from build123d import *

# Parameters (mm, degrees)
F1_DEPTH     = 6
F2_R         = 0.975
F3_DEPTH     = 6.001
F4_T1_DEPTH  = 6
F4_T3_DEPTH  = 6
F4_T5_DEPTH  = 13.5
F4_T7_DEPTH  = 13.5
F4_T9_DEPTH  = 13.5
F4_T11_DEPTH = 13.5
F4_T13_DEPTH = 13.4624057783
F5_SIZE      = 0.5


# Not quite as in the source:
# - a fillet or chamfer that OpenCascade refuses, or shapes differently, is made with other operations: its cross-section is extruded or revolved along the edge and cut away or added


with BuildPart() as f1:
    # F0 (on Top) → F1 (new body)
    with BuildSketch(Plane.XY):
        Polygon((0, 1.9), (0, 0), (1.35, 0), (1.35, 11.3), (-7.85, 11.3), (-7.85, 7.55), (-4.85, 7.55), (-4.85, 0), (-3.5, 0), (-3.5, 8.5), (0, 8.5), align=None)
        Polygon((-0.9, 0), (0, 0), (0, 1.9), (-0.9, 1), align=None)
    extrude(amount=F1_DEPTH)

    # F2 (on face) → F3 (cut, through all)
    with BuildSketch(Plane.XY.offset(6)):
        with Locations((-5.8098790534, 9.425)):
            Circle(F2_R)
    extrude(amount=-F3_DEPTH, mode=Mode.SUBTRACT)

    # F4: fillet of radius 1.5 on 7 edges, made by hand

    # F4_s2 → F4_t1 (join)
    with BuildSketch(Plane.XY):
        with BuildLine():
            ThreePointArc((0, 7), (-0.4393398282, 8.0606601718), (-1.5, 8.5))
            Line((-1.5, 8.5), (0, 8.5))
            Line((0, 8.5), (0, 7))
        make_face()
    extrude(amount=F4_T1_DEPTH)

    # F4_s4 → F4_t3 (join)
    with BuildSketch(Plane.XY):
        with BuildLine():
            ThreePointArc((-2, 8.5), (-3.0606601718, 8.0606601718), (-3.5, 7))
            Line((-3.5, 7), (-3.5, 8.5))
            Line((-3.5, 8.5), (-2, 8.5))
        make_face()
    extrude(amount=F4_T3_DEPTH)

    # F4_s6 → F4_t5 (cut)
    with BuildSketch(Plane.XY.offset(-3.75)):
        with BuildLine():
            ThreePointArc((1.35, 1.5), (0.9106601718, 0.4393398282), (-0.15, 0))
            Line((-0.15, 0), (1.35, 0))
            Line((1.35, 0), (1.35, 1.5))
        make_face()
    extrude(amount=F4_T5_DEPTH, mode=Mode.SUBTRACT)

    # F4_s8 → F4_t7 (cut)
    with BuildSketch(Plane.XY.offset(-3.75)):
        with BuildLine():
            ThreePointArc((1.35, 9.8), (0.9106601718, 10.8606601718), (-0.15, 11.3))
            Line((-0.15, 11.3), (1.35, 11.3))
            Line((1.35, 11.3), (1.35, 9.8))
        make_face()
    extrude(amount=F4_T7_DEPTH, mode=Mode.SUBTRACT)

    # F4_s10 → F4_t9 (cut)
    with BuildSketch(Plane.XY.offset(-3.75)):
        with BuildLine():
            ThreePointArc((-7.85, 9.8), (-7.4106601718, 10.8606601718), (-6.35, 11.3))
            Line((-6.35, 11.3), (-7.85, 11.3))
            Line((-7.85, 11.3), (-7.85, 9.8))
        make_face()
    extrude(amount=F4_T9_DEPTH, mode=Mode.SUBTRACT)

    # F4_s12 → F4_t11 (cut)
    with BuildSketch(Plane.XY.offset(-3.75)):
        with BuildLine():
            ThreePointArc((-6.35, 7.55), (-7.4106601718, 7.9893398282), (-7.85, 9.05))
            Line((-7.85, 9.05), (-7.85, 7.55))
            Line((-7.85, 7.55), (-6.35, 7.55))
        make_face()
    extrude(amount=F4_T11_DEPTH, mode=Mode.SUBTRACT)

    # F4_s14 → F4_t13 (cut)
    with BuildSketch(Plane.XY.offset(-3.7312028891)):
        with BuildLine():
            ThreePointArc((-3.5, 0), (-4.4624297731, 0.4862505658), (-4.85, 1.4924811557))
            Line((-4.85, 1.4924811557), (-4.85, 0))
            Line((-4.85, 0), (-3.5, 0))
        make_face()
    extrude(amount=F4_T13_DEPTH, mode=Mode.SUBTRACT)

    # F5
    f5_edges = [f1.edges().sort_by_distance(p)[0] for p in [
        (-6.784879, 9.425, 6),
        (-6.784879, 9.425, 0),
    ]]
    chamfer(f5_edges, length=F5_SIZE)


solid = f1.part
Can you work these out from the model? Positions are in its coordinate system, mm. A direction names the side the tool comes from. Round coordinates to 2 decimals unless told otherwise and drop trailing zeros. Loops run counter-clockwise (first coordinate to the right, second up) from the corner with the lowest first, then second, coordinate; pieces in that order, holes last. Notation, with made-up numbers: (2.25, 11) - (41.25, 11) arc R19 cw to (41.25, 35) - close; hole circle Ø10 at (47.5, 22). An arc over 180 degrees is marked (long way). Answer in a Markdown table with one row per item. Add a question column.
Q1. For pin 1 Ø1.2 at (x, z) = (-6, 2) entering from -Y; pin 2 Ø1.2 at (x, y) = (-5.81, 9.43) entering from -Z; pin 3 Ø1 at (x, z) = (-2.5, 3.5) entering from -Y; pin 4 Ø3 at (y, z) = (3.5, 2.5) entering from -X, each with a flat end and sliding along its axis, tell me the tip position at first contact or that it passes through.
Q2. We'd pull the mould along X, two halves only. Please class faces 1 (the cylindrical face through (-3.05, 8.07, 2.96)), 2 (the flat face through (-3.5, 3, 3)), 3 (the flat face through (-4.85, 5, 3)), 4 (the flat face through (-3.2, 8.2, 6)): pulls with the +X half, pulls with the -X half, needs draft (parallel to the pull), parting line crosses it, or undercut.
Q3. I want a section at B-B on z = 3.45. List the corners of the cut face in (x, y) for me (3 decimals).
Q4. I want a section at A-A on y = 6.25. List the corners of the cut face in (x, z) for me.
Q5. I want a section at D-D on y = 7.75. List the corners of the cut face in (x, z) for me, and give its area (3 significant figures).
Q6. Which directions (+Z, -Z, +X, -X, +Y, -Y) give clear straight access to the entire face, cutting with the end or side of a thin tool? Please do faces 5 (the cylindrical face through (-0.43, 8.05, 2.96)), 6 (the flat face through (-6, 7.55, 3)), 7 (the flat face through (-0.9, 0.5, 3)).
Q7. I need wall thicknesses on L1, parallel to X at y = 3.5, z = 2.6; L2, parallel to X at y = 1.75, z = 3.9; L3, parallel to Y at x = -0.5, z = 5.4. Which ranges of each line are inside material? Lowest first, please.
Q8. I want a section at C-C on x = 0.75. List the corners of the cut face in (y, z) for me, and give its area (3 significant figures).
A:
| question | item | result |
|---|---|---|
| 1 | pin 1 | y = 7.55 |
| 1 | pin 2 | through |
| 1 | pin 3 | y = 8.12 |
| 1 | pin 4 | x = -4.85 |
| 2 | face 1 | undercut |
| 2 | face 2 | undercut |
| 2 | face 3 | pulls with the -X half |
| 2 | face 4 | needs draft |
| 3 | outline | (-7.85, 9.05) arc R1.5 ccw to (-6.35, 7.55) - (-4.85, 7.55) - (-4.85, 1.492) arc R1.5 ccw to (-3.5, 0) - (-3.5, 7) arc R1.5 cw to (-2, 8.5) - (-1.5, 8.5) arc R1.5 cw to (0, 7) - (0, 1.9) - (-0.9, 1) - (-0.9, 0) - (-0.15, 0) arc R1.5 ccw to (1.35, 1.5) - (1.35, 9.8) arc R1.5 ccw to (-0.15, 11.3) - (-6.35, 11.3) arc R1.5 ccw to (-7.85, 9.8) - close; hole circle Ø1.95 at (-5.81, 9.425) |
| 4 | outline | (-4.85, 0) - (-3.5, 0) - (-3.5, 6) - (-4.85, 6) - close; (0, 0) - (1.35, 0) - (1.35, 6) - (0, 6) - close |
| 5 | outline | (-7.1, 0) - (-3.3, 0) - (-3.3, 6) - (-7.1, 6) - close; (-0.2, 0) - (1.35, 0) - (1.35, 6) - (-0.2, 6) - close |
| 5 | area | 32.1 mm^2 |
| 6 | face 5 | +Z, -Z |
| 6 | face 6 | +Z, -Z, -X, -Y |
| 6 | face 7 | +Z, -Z, -Y |
| 7 | L1 | -4.85 to -3.5, 0 to 1.35 |
| 7 | L2 | -4.85 to -3.5, -0.15 to 1.35 |
| 7 | L3 | 0 to 1.4, 8.12 to 11.3 |
| 8 | outline | (0.3, 0) - (11, 0) - (11, 6) - (0.3, 6) - close |
| 8 | area | 64.2 mm^2 |
